```python
from build123d import *

# Parameters (mm, degrees)
PAD031_DEPTH = 1.4
SKETCH158_W  = 1.8
SKETCH158_H  = 16
PAD032_DEPTH = 6.4
SKETCH159_W  = 1.6
SKETCH159_H  = 4.4
PAD033_DEPTH = 1.4


with BuildPart() as part:
    # Sketch157 → Pad031 (new body)
    with BuildSketch(Plane.XY):
        Polygon((1.8, 8), (17, 8), (17, 6), (19, 6), (19, -6), (17, -6), (17, -8), (1.8, -8), (0, -8), (0, 8), align=None)
    extrude(amount=PAD031_DEPTH)

    # Sketch158 (on Face8 of Pad031) → Pad032 (join)
    with BuildSketch(Plane.XY.offset(1.4)):
        with Locations((0.9, 0)):
            Rectangle(SKETCH158_W, SKETCH158_H)
    extrude(amount=PAD032_DEPTH)

    # Sketch159 (on Face9 of Pad032) → Pad033 (join)
    with BuildSketch(Plane.XY.offset(7.8)):
        with Locations((0.9, 0)):
            Rectangle(SKETCH159_W, SKETCH159_H)
    extrude(amount=PAD033_DEPTH)


solid = part.part
```
Design review of the part built by this model. Coordinates are the model's own, in mm. A direction names the side the tool comes from. Give positions to 0.01 mm unless a question says otherwise; leave off trailing zeros. Write each loop counter-clockwise with the first axis right and the second up, starting at its lowest first coordinate (ties: lowest second). Pieces come first, ordered by that corner, then holes. Notation, with made-up numbers: (46.25, -9.75) - (84.25, -9.75) arc R20 ccw to (84.25, -0.75) - close; hole circle Ø9 at (10.5, -15). An arc over 180 degrees is marked (long way). Return JSON: item names as keys, results as strings. Group by question number.
(1) We need section B-B, the plane x = 10.25. Give the boundary of the cut face in (y, z), then the cut area to 3 significant figures.
(2) Insertion check: pin 1 (5 mm diameter, centred on y = -4, z = 7.5, fed in from +X); pin 2 (1.1 mm diameter, centred on x = 1, z = 8.5, fed in from -Y); pin 3 (0.7 mm diameter, centred on y = 7.5, z = 1, fed in from +X). Each pin has a flat end and moves straight along its axis. Give the tip position at first contact, or say it passes through.
(3) We need section C-C, the plane z = 4.5. Give the boundary of the cut face in (x, y), then the cut area to 3 significant figures.
(4) We need section A-A, the plane y = -1.25. Give the boundary of the cut face in (x, z), then the cut area to 3 significant figures.
(5) To check wall thickness, follow probe 1 along Z at (x, y) = (3.5, 3.5); probe 2 along X at (y, z) = (7.75, 2.5); probe 3 along X at (y, z) = (6.25, 1). State the ranges of each line that lie inside material, in increasing order.
(6) Machinability: for faces 1 (the flat face through (17, -7, 1)), 2 (the flat face through (0.1, 0, 8)), 3 (the flat face through (1, -2.2, 8)), 4 (the flat face through (1.8, 0, 5)), 5 (the flat face through (18, 6, 1)), which of the approach directions +Z, -Z, +X, -X, +Y, -Y give a long, thin tool a straight path to every point of the face, cutting with its end or side? Answer none if there is none.
(7) We need section D-D, the plane y = 4. Give the boundary of the cut face in (x, z), then the cut area to 3 significant figures.
Reported:
{
 "1": {"outline": "(-8, 0) - (8, 0) - (8, 1.4) - (-8, 1.4) - close", "area": "22.4 mm2"},
 "2": {"pin 1": "stops at x = 1.8", "pin 2": "stops at y = -2.2", "pin 3": "stops at x = 17"},
 "3": {"outline": "(0, -8) - (1.8, -8) - (1.8, 8) - (0, 8) - close", "area": "28.8 mm2"},
 "4": {"outline": "(0, 0) - (19, 0) - (19, 1.4) - (1.8, 1.4) - (1.8, 7.8) - (1.7, 7.8) - (1.7, 9.2) - (0.1, 9.2) - (0.1, 7.8) - (0, 7.8) - close", "area": "40.4 mm2"},
 "5": {"probe 1": "z = 0 to 1.4", "probe 2": "x = 0 to 1.8", "probe 3": "x = 0 to 17"},
 "6": {"face 1": "+Z, -Z, +X, -Y", "face 2": "+Z, -X, +Y, -Y", "face 3": "+Z, +X, -X, -Y", "face 4": "+Z, +X, +Y, -Y", "face 5": "+Z, -Z, +X, +Y"},
 "7": {"outline": "(0, 0) - (19, 0) - (19, 1.4) - (1.8, 1.4) - (1.8, 7.8) - (0, 7.8) - close", "area": "38.1 mm2"}
}
